Autodesk Inventor part; units mm, degrees
ref_plane "YZ Plane" through (0, 0, 0) normal (1, 0, 0) x (0, 1, 0)
ref_plane "XZ Plane" through (0, 0, 0) normal (0, 1, 0) x (-1, 0, 0)
ref_plane "XY Plane" through (0, 0, 0) normal (0, 0, 1) x (1, 0, 0)
sketch "Skizze1" plane through (0, 0, 0) normal (1, 0, 0) x (0, 1, 0)
  circle A0 centre (0, 0) radius 3
  line L0 (1.4434, 0) -> (0.7217, -1.25)
  line L1 (0.7217, -1.25) -> (-0.7217, -1.25)
  line L2 (-0.7217, -1.25) -> (-1.4434, 0)
  line L3 (-1.4434, 0) -> (-0.7217, 1.25)
  line L4 (-0.7217, 1.25) -> (0.7217, 1.25)
  line L5 (0.7217, 1.25) -> (1.4434, 0)
  point P0 (0, -1.25)
  point P1 (0, 1.25)
  dimension "d0" = 6
  dimension "d1" = 2.5
extrude "Extrusion1" add sketch "Skizze1" along normal blind 6
sketch "Skizze2" plane through (0, 0, 0) normal (-1, 0, 0) x (0, 0, 1)
  circle A0 centre (0, 0) radius 3
  line L0 (0, 1.4434) -> (-1.25, 0.7217)
  line L1 (1.25, 0.7217) -> (0, 1.4434)
  line L2 (1.25, -0.7217) -> (1.25, 0.7217)
  line L3 (0, -1.4434) -> (1.25, -0.7217)
  line L4 (-1.25, -0.7217) -> (0, -1.4434)
  line L5 (-1.25, 0.7217) -> (-1.25, -0.7217)
  circle A1 centre (0, 0) radius 3
extrude "Extrusion2" add sketch "Skizze2" along normal blind 5 contours A0 | L1 L2 L3 L4 L5 L0
chamfer "Fase1" distance 1 angle 45 6 edges at (6, 1.0825, 0.625) (6, 1.0825, -0.625) (6, 0, -1.25) (6, -1.0825, -0.625) (6, -1.0825, 0.625) (6, 0, 1.25)
properties part number "40_XYZstage_micrometer_motorized_nema8_zadapter_m2.5nut"
Read the model definition and answer for the solid it produces. Units are mm, in the model's axes. A direction names the side the tool comes from. Give positions to 0.01 mm unless a question says otherwise; leave off trailing zeros. Order: outer loops, then holes, each group sorted by start corner. A loop starts at its lowest first (then second) coordinate and runs counter-clockwise, first axis right, second up.
(1) Find section A-A (x = 4.5). Give the vertices of the cut face in (y, z), plus the area to 3 significant figures.
(2) Given pin 1 (2 mm diameter, centred on x = -1.5, z = 1.5, fed in from +Y); pin 2 (0.8 mm diameter, centred on y = -0.5, z = 0, fed in from +X), each flat-ended and moving along its own axis, determine where each tip first touches the part or whether it passes through.
(3) Find section C-C (x = -1.5). Give the vertices of the cut face in (y, z).
(4) Straight lines are drawn through the part: L1, parallel to X at y = 0.3, z = 0.35; L2, parallel to Z at x = 4.25, y = 0.1; L3, parallel to Z at x = 1, y = 1. For each, find the intervals that lie inside material, in ascending order.
(5) For a pull along Z with two mould halves and no side action, classify faces 1 (the flat face through (2.465, 1.088, -0.616)), 2 (the cylindrical face through (-0.799, 1.117, 2.784)), 3 (the flat face through (-5, 0, 0)) as released by +Z, released by -Z, zero draft, split by the parting line, or undercut.
(6) For faces 4 (the flat face through (5.5, 1.5, -0.9)), 5 (the flat face through (6, 2, -2)), determine the directions among +Z, -Z, +X, -X, +Y, -Y from which every point of the face is accessible in a straight line to the end or side of a thin tool.
(7) Find section B-B (z = -0.35). Give the vertices of the cut face in (x, y), plus the area to 3 significant figures.
Result sheet:
1. outline: circle Ø6 at (0, 0); hole (-1.44, 0) - (-0.72, -1.25) - (0.72, -1.25) - (1.44, 0) - (0.72, 1.25) - (-0.72, 1.25) - close
1. area: 22.9 mm2
2. pin 1: stops at y = 2.96
2. pin 2: stops at x = 0
3. outline: circle Ø6 at (0, 0)
4. L1: x = -5 to 0
4. L2: z = -3 to -1.25, 1.25 to 3
4. L3: z = -2.83 to -0.77, 0.77 to 2.83
5. face 1: undercut
5. face 2: split by the parting line
5. face 3: zero draft
6. face 4: +X
6. face 5: +Z, -Z, +X, +Y, -Y
7. outline: (-5, -2.98) - (6, -2.98) - (6, -2.4) - (5, -1.24) - (0, -1.24) - (0, 1.24) - (5, 1.24) - (6, 2.4) - (6, 2.98) - (-5, 2.98) - close
7. area: 49.5 mm2
